from build123d import *

# Parameters (mm, degrees)
SKETCH1_R           = 15
SKETCH1_R_2         = 8.5
BOSS_EXTRUDE1_DEPTH = 7
CHAMFER1_SIZE       = 0.5
SKETCH2_R           = 13.85
SKETCH2_R_2         = 9.7
CUT_EXTRUDE1_DEPTH  = 0.5
SKETCH3_R           = 13.85
SKETCH3_R_2         = 9.7
CUT_EXTRUDE2_DEPTH  = 0.5


with BuildPart() as part:
    # Sketch1 → Boss-Extrude1 (new body)
    with BuildSketch(Plane(origin=(0, 0, 0), x_dir=(0, 0, -1), z_dir=(1, 0, 0))):
        Circle(SKETCH1_R)
        Circle(SKETCH1_R_2, mode=Mode.SUBTRACT)
    extrude(amount=BOSS_EXTRUDE1_DEPTH)

    # Chamfer1
    chamfer1_edges = [part.edges().sort_by_distance(p)[0] for p in [
        (0, 0, 15),
        (7, 0, 15),
        (0, 0, 8.5),
        (7, 0, 8.5),
    ]]
    chamfer(chamfer1_edges, length=CHAMFER1_SIZE)

    # Sketch2 → Cut-Extrude1 (cut)
    with BuildSketch(Plane(origin=(7, 0, 0), x_dir=(0, 0, -1), z_dir=(1, 0, 0))):
        Circle(SKETCH2_R)
        Circle(SKETCH2_R_2, mode=Mode.SUBTRACT)
    extrude(amount=-CUT_EXTRUDE1_DEPTH, mode=Mode.SUBTRACT)

    # Sketch3 → Cut-Extrude2 (cut)
    with BuildSketch(Plane.ZY):
        Circle(SKETCH3_R)
        Circle(SKETCH3_R_2, mode=Mode.SUBTRACT)
    extrude(amount=-CUT_EXTRUDE2_DEPTH, mode=Mode.SUBTRACT)


solid = part.part
The listing builds one solid part. Answer for the finished solid, in the listing's coordinates (mm). A direction names the side the tool comes from. Round coordinates to 2 decimals unless told otherwise and drop trailing zeros. Loops run counter-clockwise (first coordinate to the right, second up) from the corner with the lowest first, then second, coordinate; pieces in that order, holes last. Notation, with made-up numbers: M -7.75,-21 L 6.25,-21 A20 cw 6.25,-7 Z; hole C -33,71 d9. An arc over 180 degrees is marked long. Return JSON: item names as keys, results as strings.
Q1. Find the intervals of material crossed by line 1 along Y through (x, z) = (4.85, 0); line 2 along Y through (x, z) = (0.45, 0); line 3 along Y through (x, z) = (6.6, 0), in increasing order. Write a range as from..to.
Results list:
{"line 1": "y = -15..-8.5, 8.5..15", "line 2": "y = -14.95..-13.85, -9.7..-8.55, 8.55..9.7, 13.85..14.95", "line 3": "y = -14.9..-13.85, -9.7..-8.6, 8.6..9.7, 13.85..14.9"}
Q2. The mould has two halves that part along Z. Classify faces 4 (the face through (0, -14, -1)), 5 (the face through (3.458, 0.66, 14.985)), 6 (the face through (0.25, 4.16, 13.21)): released by +Z, released by -Z, zero draft, split by the parting line, or undercut.
Results list:
{"face 4": "zero draft", "face 5": "split by the parting line", "face 6": "undercut"}
Q3. Each of these flat-tipped pins is pushed along its axis until it touches: pin 1 Ø2 at (x, y) = (4.5, 10) entering from -Z; pin 2 Ø2 at (x, z) = (1, -11.5) entering from -Y. Where does it stop, or does it pass through?
Results list:
{"pin 1": "stops at z = -12", "pin 2": "stops at y = -10.71"}
Q4. Which of the six approach directions +Z, -Z, +X, -X, +Y, -Y give full straight-line access (tool end or side, diameter ignored) to faces 1 (the face through (3.458, 7.167, -4.57)), 2 (the face through (6.5, 9.43, -2.88)), 3 (the face through (0.5, 9.43, 2.88))?
Results list:
{"face 1": "+X, -X", "face 2": "+X", "face 3": "-X"}
Q5. Find section C-C, the plane x = 4.5. Determine the outline of the cut face in (y, z), plus the area to 3 significant figures.
Results list:
{"outline": "C 0,0 d30; hole C 0,0 d17", "area": "480 mm2"}
